Check sheet for the drawn part. Datum: minimum x, y, z corner. Units: mm. A direction names the side the tool comes from. Give positions to 0.01 mm unless a question says otherwise; leave off trailing zeros. Loops run counter-clockwise (first coordinate to the right, second up) from the corner with the lowest first, then second, coordinate; pieces in that order, holes last. Notation, with made-up numbers: (-3.5, 55.5) - (41.5, 55.5) arc R24 cw to (41.5, 74.5) - close; hole circle Ø11 at (-22.5, -1.5). An arc over 180 degrees is marked (long way). One line per item, written item: value. Start each with the question number.
1. Gauge pin test, flat ends, axial feed: pin 1 (3 mm diameter, centred on x = 10.5, y = 16, fed in from -Z); pin 2 (1.5 mm diameter, centred on x = 32.5, z = 3, fed in from -Y). Record the tip position at first contact, or that the pin passes through.
2. Access from +Z, -Z, +X, -X, +Y, -Y to the whole of each face (thin tool, end or side, straight path). Record for the marked faces 1, 2, 3 and 4.
3. Sectioned sample at D-D (y = 8.25). Record the cut outline in (x, z).
4. Sectioned sample at C-C (x = 58). Record the cut outline in (y, z).
5. Scan lines: L1, parallel to Y at x = 46.95, z = 3.5; L2, parallel to Y at x = 16, z = 2; L3, parallel to X at y = 19.25, z = 2. Record each from-to range of solid material in increasing order. Write a range as [from, to].
6. Sectioned sample at B-B (y = 5.5). Record the cut outline in (x, z).
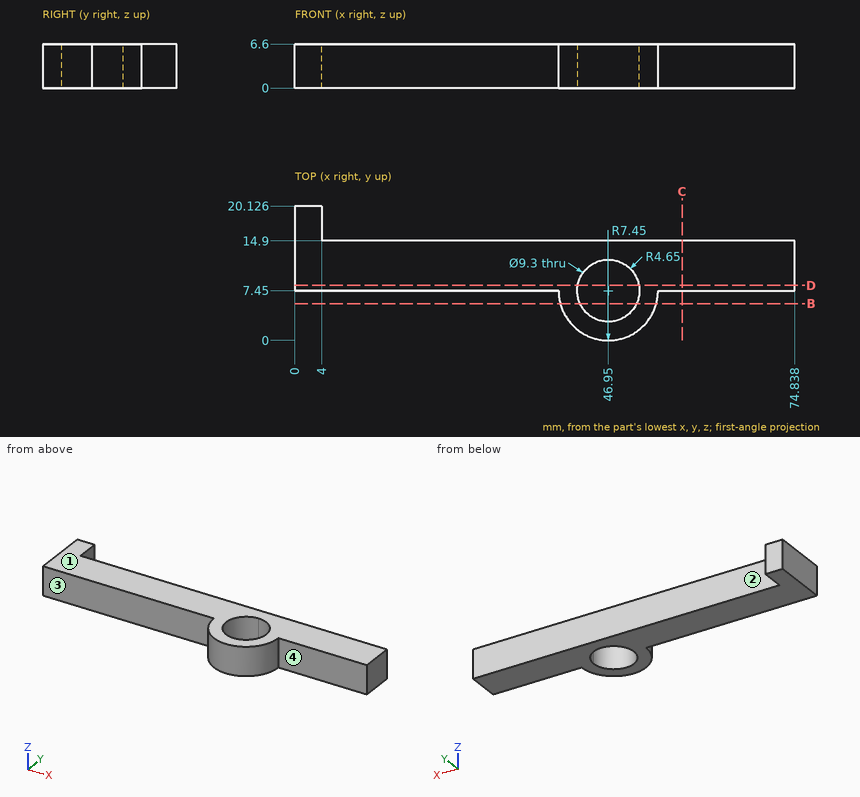
Results are:
1. pin 1: stops at z = 0
1. pin 2: stops at y = 7.45
2. face 1: +Z, +X, -X, +Y, -Y
2. face 2: +Z, -Z, +X, +Y
2. face 3: +Z, -Z, -X, -Y
2. face 4: +Z, -Z, +X, -Y
3. outline: (0, 0) - (42.37, 0) - (42.37, 6.6) - (0, 6.6) - close; (51.53, 0) - (74.84, 0) - (74.84, 6.6) - (51.53, 6.6) - close
4. outline: (7.45, 0) - (14.9, 0) - (14.9, 6.6) - (7.45, 6.6) - close
5. L1: y = [0, 2.8], [12.1, 14.9]
5. L2: y = [7.45, 14.9]
5. L3: x = [0, 4]
6. outline: (39.76, 0) - (42.73, 0) - (42.73, 6.6) - (39.76, 6.6) - close; (51.17, 0) - (54.14, 0) - (54.14, 6.6) - (51.17, 6.6) - close
